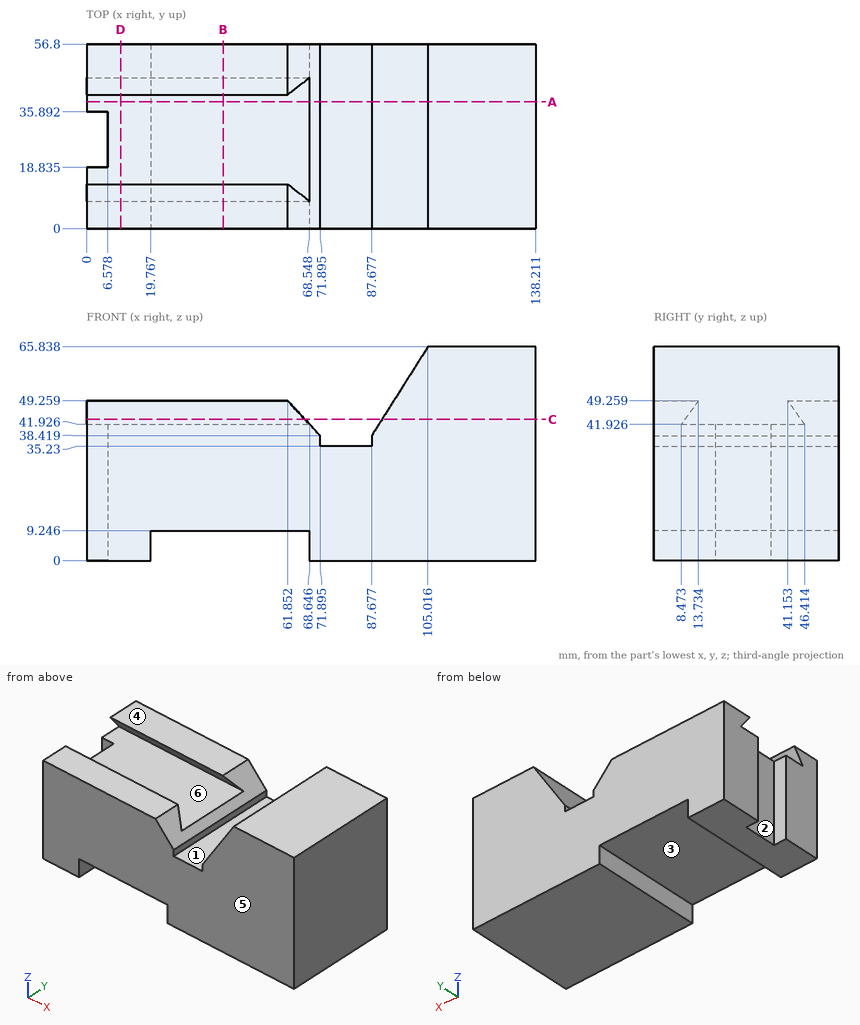
The figure shows three views and two pictorial views of one solid part (mm, origin at its lowest corner). Answer the questions. A direction names the side the tool comes from. Coordinates: 2 decimals unless noted, no trailing zeros. Write each loop counter-clockwise with the first axis right and the second up, starting at its lowest first coordinate (ties: lowest second). Pieces come first, ordered by that corner, then holes. Notation, with made-up numbers: (68.25, 2.25) -> (111.25, 2.25) arc R23 ccw to (111.25, 23.25) -> close; hole circle Ø1 at (37, 51). An arc over 180 degrees is marked (long way). Return JSON: item names as keys, results as strings.
1. A cutting plane is placed at C-C (z = 43.5). Determine the outline of the cut face in (x, y) (1 decimal), and give its area (3 significant figures).
Found:
{"outline": "(0, 0) -> (67.2, 0) -> (67.2, 9.6) -> (0, 9.6) -> close; (0, 45.3) -> (67.2, 45.3) -> (67.2, 56.8) -> (0, 56.8) -> close; (90.9, 0) -> (138.2, 0) -> (138.2, 56.8) -> (90.9, 56.8) -> close", "area": "4,110 mm2"}
2. A tool of negligible diameter and unlimited length cuts with its end or side. For the marked faces 1, 2 and 3, from which of +Z, -Z, +X, -X, +Y, -Y can it reach the whole face along a straight path? Write none if from no direction.
Found:
{"face 1": "+Z, +Y, -Y", "face 2": "+Z, -Z, -X", "face 3": "-Z, +Y, -Y"}
3. Each of these flat-tipped pins is pushed along its axis until it touches: P1, Ø8.5, axis at y = 26, z = 17, coming from the -X side; P2, Ø4.5, axis at x = 43, y = 51.5, coming from the +Z side; P3, Ø8, axis at x = 21, y = 32.5, coming from the +Z side. Where does it stop, or does it pass through?
Found:
{"P1": "x = 6.58", "P2": "z = 49.26", "P3": "z = 41.93"}
4. Find the intervals of material crossed by line 1 along X through (y, z) = (43, 35.5) (1 decimal); line 2 along X through (y, z) = (23.5, 8); line 3 along Z through (x, y) = (67, 35.5) (1 decimal), in increasing order. Write a range as from..to.
Found:
{"line 1": "0..71.9, 87.7..138.2", "line 2": "6.58..19.77, 68.55..138.21", "line 3": "9.2..41.9"}
5. A cutting plane is placed at D-D (x = 10.5). Determine the outline of the cut face in (y, z) (1 decimal).
Found:
{"outline": "(0, 0) -> (56.8, 0) -> (56.8, 49.3) -> (41.2, 49.3) -> (46.4, 41.9) -> (8.5, 41.9) -> (13.7, 49.3) -> (0, 49.3) -> close"}
6. Determine the mould class of the marked faces 4, 5 and 6 for opening direction Y: pulls with the +Y half, pulls with the -Y half, needs draft (parallel to the pull), parting line crosses it, or undercut.
Found:
{"face 4": "needs draft", "face 5": "pulls with the -Y half", "face 6": "undercut"}
7. A cutting plane is placed at B-B (x = 42). Determine the outline of the cut face in (y, z) (1 decimal), and give its area (3 significant figures).
Found:
{"outline": "(0, 9.2) -> (56.8, 9.2) -> (56.8, 49.3) -> (41.2, 49.3) -> (46.4, 41.9) -> (8.5, 41.9) -> (13.7, 49.3) -> (0, 49.3) -> close", "area": "2,030 mm2"}
8. A cutting plane is placed at A-A (y = 39). Determine the outline of the cut face in (x, z) (1 decimal), and give its area (3 significant figures).
Found:
{"outline": "(0, 0) -> (19.8, 0) -> (19.8, 9.2) -> (68.5, 9.2) -> (68.5, 0) -> (138.2, 0) -> (138.2, 65.8) -> (105, 65.8) -> (87.7, 38.4) -> (87.7, 35.2) -> (71.9, 35.2) -> (71.9, 38.4) -> (68.6, 41.9) -> (0, 41.9) -> close", "area": "6,200 mm2"}
